Could you check a few things on this drawing? It's one solid part, dimensions in mm from its lowest x, y, z. A direction names the side the tool comes from. Round coordinates to 2 decimals unless told otherwise and drop trailing zeros. Order: outer loops, then holes, each group sorted by start corner. A loop starts at its lowest first (then second) coordinate and runs counter-clockwise, first axis right, second up. Notation, with made-up numbers: (35, -16.5) - (50, -16.5) arc R27 cw to (50, 19.5) - close; hole circle Ø10 at (13, -19.75). An arc over 180 degrees is marked (long way). Use one line per item in the form item = value.
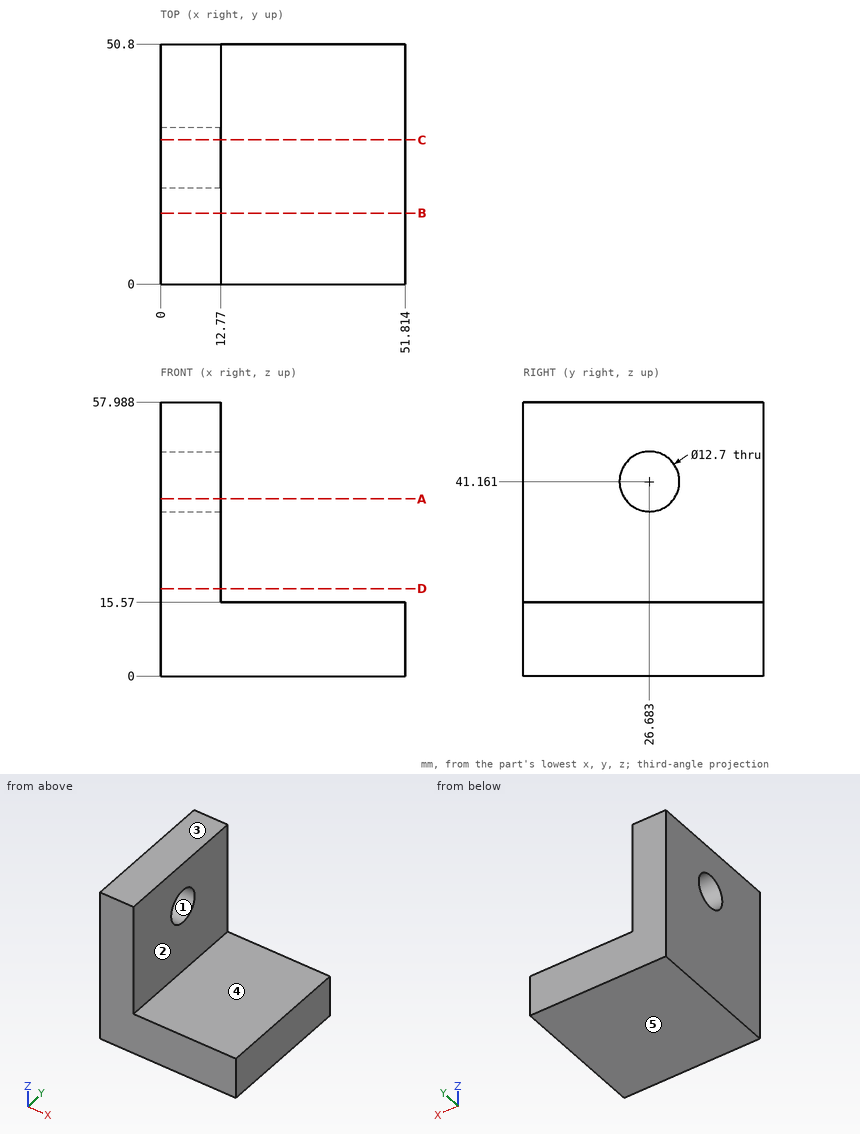
Item 1: I need wall thicknesses on L1, parallel to X at y = 44, z = 56; L2, parallel to Z at x = 38, y = 6.5; L3, parallel to Y at x = 5, z = 46 (1 decimal). Which ranges of each line are inside material? Lowest first, please.
Found:
L1 = 0 to 12.77
L2 = 0 to 15.57
L3 = 0 to 22.6, 30.8 to 50.8
Item 2: Imagine slicing it at D-D on z = 18.5. Please give me the cut outline in (x, y).
Found:
outline = (0, 0) - (12.77, 0) - (12.77, 50.8) - (0, 50.8) - close
Item 3: For the marked faces 4 and 5, which set-ups out of +Z, -Z, +X, -X, +Y, -Y let a thin tool reach every point of the face, with its end or its side?
Found:
face_4 = +Z, +X, +Y, -Y
face_5 = -Z, +X, -X, +Y, -Y
Item 4: Will these pins go through, and if not, where does the flat tip stop? P1, Ø21, axis at y = 16.5, z = 33, coming from the +X side; P2, Ø10, axis at y = 26.68, z = 41.16, coming from the +X side; P3, Ø1, axis at x = 17.5, y = 45, coming from the +Z side.
Found:
P1 = 12.77
P2 = through
P3 = 15.57
Item 5: Imagine slicing it at C-C on y = 30.5. Please give me the cut outline in (x, z) (1 decimal), plus the area to 3 significant figures.
Found:
outline = (0, 0) - (51.8, 0) - (51.8, 15.6) - (12.8, 15.6) - (12.8, 36.1) - (0, 36.1) - close; (0, 46.2) - (12.8, 46.2) - (12.8, 58) - (0, 58) - close
area = 1,220 mm2
Item 6: Imagine slicing it at A-A on z = 37.5. Please give me the cut outline in (x, y) (1 decimal), plus the area to 3 significant figures.
Found:
outline = (0, 0) - (12.8, 0) - (12.8, 21.5) - (0, 21.5) - close; (0, 31.9) - (12.8, 31.9) - (12.8, 50.8) - (0, 50.8) - close
area = 516 mm2
Item 7: If we mould it in two halves opening along Z, with no side actions, what happens to the marked faces 1, 2 and 3? For each: released by +Z, released by -Z, zero draft, split by the parting line, or undercut.
Found:
face_1 = undercut
face_2 = zero draft
face_3 = released by +Z
Item 8: Imagine slicing it at B-B on y = 15. Please give me the cut outline in (x, z).
Found:
outline = (0, 0) - (51.81, 0) - (51.81, 15.57) - (12.77, 15.57) - (12.77, 57.99) - (0, 57.99) - close
